Could you check a few things on this model? Use its own coordinates, in mm. Face numbers are marked on the shaded views. A direction names the side the tool comes from. Give positions to 0.01 mm unless a question says otherwise; leave off trailing zeros. Write each loop counter-clockwise with the first axis right and the second up, starting at its lowest first coordinate (ties: lowest second). Pieces come first, ordered by that corner, then holes. Notation, with made-up numbers: (84.5, 39) - (141.5, 39) arc R21 ccw to (141.5, 47) - close; hole circle Ø8 at (18, 8.25). An arc over 180 degrees is marked (long way). Write item = value, one per line.
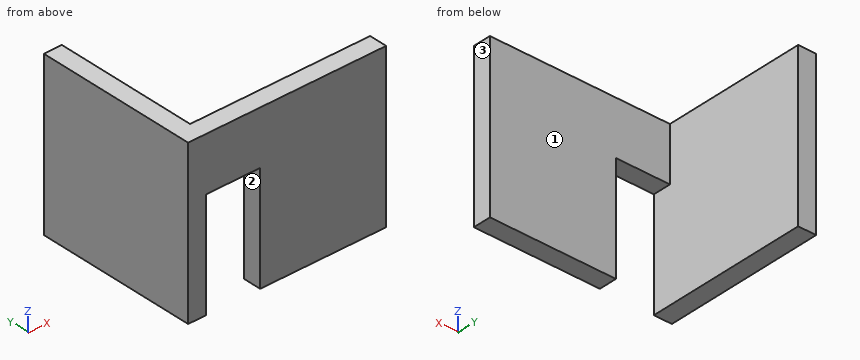
from build123d import *

# Parameters (mm, degrees)
BOX012_W     = 1
BOX012_H     = 9
BOX012_DEPTH = 9
BOX011_W     = 7
BOX011_H     = 1
BOX011_DEPTH = 9
BOX013_W     = 3
BOX013_H     = 1
BOX013_DEPTH = 3


with BuildPart() as box012:
    # Box012 → Box012 (new body)
    with BuildSketch(Plane(origin=(33, 15, 1), x_dir=(1, 0, 0), z_dir=(0, 0, 1))):
        with Locations((0.5, 4.5)):
            Rectangle(BOX012_W, BOX012_H)
    extrude(amount=BOX012_DEPTH)


with BuildPart() as box011:
    # Box011 → Box011 (new body)
    with BuildSketch(Plane(origin=(37, 15, 1), x_dir=(1, 0, 0), z_dir=(0, 0, 1))):
        with Locations((3.5, 0.5)):
            Rectangle(BOX011_W, BOX011_H)
    extrude(amount=BOX011_DEPTH)


with BuildPart() as fusion003:
    # Box013 → Box013 (new body)
    with BuildSketch(Plane(origin=(34, 15, 7), x_dir=(1, 0, 0), z_dir=(0, 0, 1))):
        with Locations((1.5, 0.5)):
            Rectangle(BOX013_W, BOX013_H)
    extrude(amount=BOX013_DEPTH)

    # Fusion003: union Box012, Box011
    add(box012.part)
    add(box011.part)


with BuildPart() as fusion003_1:
    # Fusion003 placement: moved
    add(fusion003.part.moved(Location((-7, 0, 0))))


solid = fusion003_1.part
1. If we section it at B-B, the plane y = 20.5: Please give me the cut outline in (x, z), and give its area (3 significant figures).
Filled sheet:
outline = (26, 1) - (27, 1) - (27, 10) - (26, 10) - close
area = 9.00 mm2
2. For pin 1 (3 mm diameter, centred on y = 20.5, z = 7.5, fed in from +X); pin 2 (4.5 mm diameter, centred on x = 34, z = 3.5, fed in from +Y), each with a flat end and sliding along its axis, tell me the tip position at first contact or that it passes through.
Filled sheet:
pin_1 = 27
pin_2 = 16
3. Which directions (+Z, -Z, +X, -X, +Y, -Y) give clear straight access to the entire face, cutting with the end or side of a thin tool? Please do the marked faces 1, 2 and 3.
Filled sheet:
face_1 = +Z, -Z, +X, +Y
face_2 = -Z, +Y, -Y
face_3 = +Z, -Z, +X, +Y, -Y
4. I need wall thicknesses on line 1 (X direction, y = 15.75, z = 3.5); line 2 (X direction, y = 20.5, z = 3.25); line 3 (Y direction, x = 27.25, z = 9). Which ranges of each line are inside material? Lowest first, please.
Filled sheet:
line_1 = 26 to 27, 30 to 37
line_2 = 26 to 27
line_3 = 15 to 16
5. If we section it at A-A, the plane z = 2: Please give me the cut outline in (x, y), and give its area (3 significant figures).
Filled sheet:
outline = (26, 15) - (27, 15) - (27, 24) - (26, 24) - close; (30, 15) - (37, 15) - (37, 16) - (30, 16) - close
area = 16.0 mm2
6. If we section it at C-C, the plane x = 28.75: Please give me the cut outline in (y, z).
Filled sheet:
outline = (15, 7) - (16, 7) - (16, 10) - (15, 10) - close
